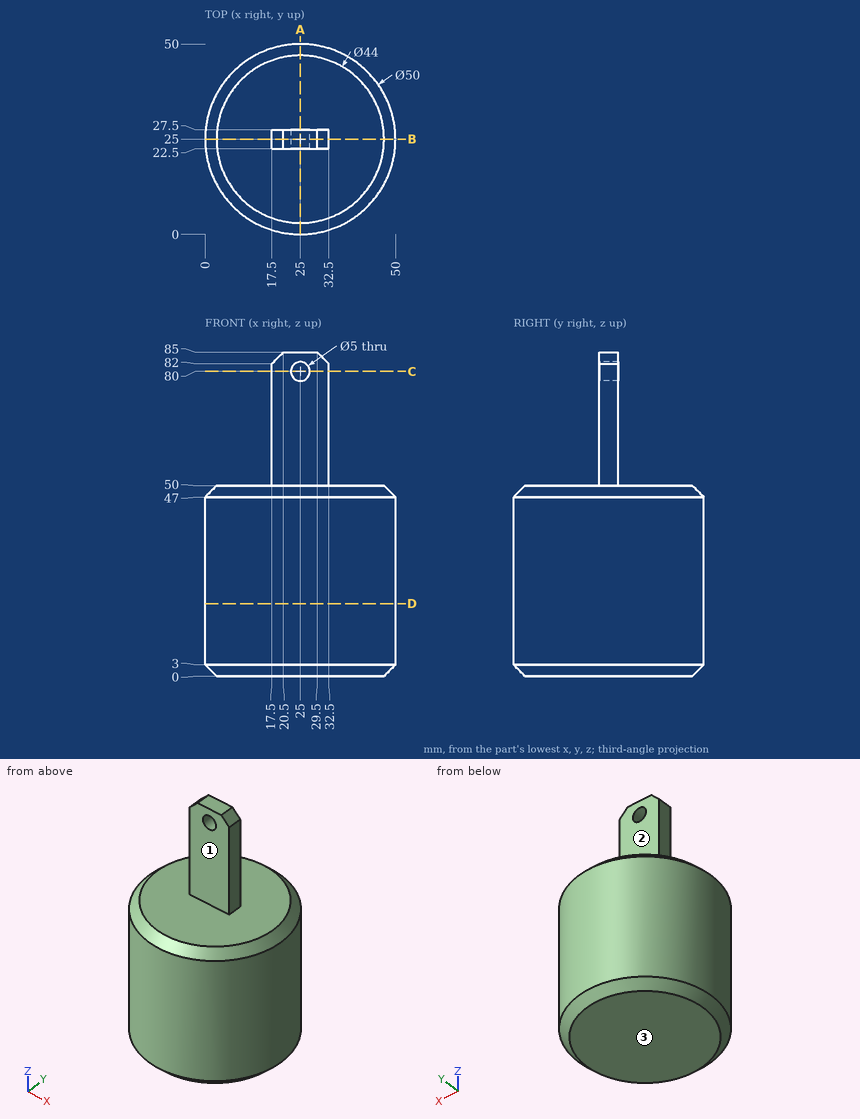
Could you check a few things on this drawing? It's one solid part, dimensions in mm from its lowest x, y, z. A direction names the side the tool comes from. Give positions to 0.01 mm unless a question says otherwise; leave off trailing zeros. Order: outer loops, then holes, each group sorted by start corner. A loop starts at its lowest first (then second) coordinate and runs counter-clockwise, first axis right, second up. Notation, with made-up numbers: M 75.25,17 L 134.25,17 A16 cw 134.25,42 Z; hole C 37.5,22.5 d1. An arc over 180 degrees is marked long. Use one line per item in the form item = value. Start each with the question number.
Item 1: If I drill on line 1 along Z through (x, y) = (25, 24); line 2 along Y through (x, z) = (26, 72); line 3 along Z through (x, y) = (11, 30), over which ranges is the centre line in solid material (lowest first)?
Item 2: If we section it at B-B (y = 25): Write out the boundary of the cut face in (x, z), then the cut area to 3 significant figures.
Item 3: Will these pins go through, and if not, where does the flat tip stop? pin 1 Ø3 at (x, z) = (31.5, 17.5) entering from +Y; pin 2 Ø2.5 at (y, z) = (24, 66) entering from +X; pin 3 Ø5 at (x, z) = (7.5, 36) entering from -Y; pin 4 Ø3 at (x, y) = (32, 10.5) entering from -Z.
Item 4: If we section it at D-D (z = 19): Write out the boundary of the cut face in (x, y), then the cut area to 3 significant figures.
Item 5: If we section it at C-C (z = 80): Write out the boundary of the cut face in (x, y), then the cut area to 3 significant figures.
Item 6: If we section it at A-A (x = 25): Write out the boundary of the cut face in (y, z).
Item 7: For the marked faces 1, 2 and 3, which set-ups out of +Z, -Z, +X, -X, +Y, -Y let a thin tool reach every point of the face, with its end or its side?
Outcome:
q1.line_1 = 0 to 77.5, 82.5 to 85
q1.line_2 = 22.5 to 27.5
q1.line_3 = 0 to 50
q2.outline = M 0,3 L 3,0 L 47,0 L 50,3 L 50,47 L 47,50 L 32.5,50 L 32.5,82 L 29.5,85 L 20.5,85 L 17.5,82 L 17.5,50 L 3,50 L 0,47 Z; hole C 25,80 d5
q2.area = 2,980 mm2
q3.pin_1 = 49.49
q3.pin_2 = 32.5
q3.pin_3 = 5
q3.pin_4 = 0
q4.outline = C 25,25 d50
q4.area = 1,960 mm2
q5.outline = M 17.5,22.5 L 22.5,22.5 L 22.5,27.5 L 17.5,27.5 Z; M 27.5,22.5 L 32.5,22.5 L 32.5,27.5 L 27.5,27.5 Z
q5.area = 50.0 mm2
q6.outline = M 0,3 L 3,0 L 47,0 L 50,3 L 50,47 L 47,50 L 27.5,50 L 27.5,77.5 L 22.5,77.5 L 22.5,50 L 3,50 L 0,47 Z; M 22.5,82.5 L 27.5,82.5 L 27.5,85 L 22.5,85 Z
q7.face_1 = +Z, +X, -X, -Y
q7.face_2 = +Z, +X, -X, +Y
q7.face_3 = -Z, +X, -X, +Y, -Y
